from build123d import *

# Parameters (mm, degrees)
SKETCH1_R               = 41.275
SKETCH1_R_2             = 18.6309
BOSS_EXTRUDE1_DEPTH     = 3.81
CUT_EXTRUDE1_DEPTH      = 59.495874641
CUT_EXTRUDE1_DEPTH_BACK = 59.495874641
SKETCH3_R               = 1.049274
CUT_EXTRUDE2_DEPTH      = 59.495874641
CUT_EXTRUDE2_DEPTH_BACK = 59.495874641
SKETCH4_R               = 1.9431


with BuildPart() as part:
    # Sketch1 → Boss-Extrude1 (new body)
    with BuildSketch(Plane(origin=(0, 0, 0), x_dir=(1, 0, 0), z_dir=(0, 1, 0))):
        with Locations(Location((0, 0, 0), (0, 0, 90))):
            Circle(SKETCH1_R)
        with Locations(Location((0, 0, 0), (0, 0, 90))):
            Circle(SKETCH1_R_2, mode=Mode.SUBTRACT)
    extrude(amount=BOSS_EXTRUDE1_DEPTH)

    # Sketch3 → Cut-Extrude1 (cut, two sides: drawn at the far end of the back side and taken through both)
    with BuildSketch(Plane.XZ.offset(-CUT_EXTRUDE1_DEPTH_BACK)):
        with Locations(Location((12.96732128, 21.997045256, 0), (0, 0, 270))):
            Circle(SKETCH3_R)
        with Locations(Location((-12.43267872, 21.997045256, 0), (0, 0, 270))):
            Circle(SKETCH3_R)
        with Locations(Location((-25.13267872, 0, 0), (0, 0, 270))):
            Circle(SKETCH3_R)
        with Locations(Location((-12.43267872, -21.997045256, 0), (0, 0, 270))):
            Circle(SKETCH3_R)
        with Locations(Location((12.96732128, -21.997045256, 0), (0, 0, 270))):
            Circle(SKETCH3_R)
        with Locations(Location((25.66732128, 0, 0), (0, 0, 270))):
            Circle(SKETCH3_R)
    extrude(amount=CUT_EXTRUDE1_DEPTH + CUT_EXTRUDE1_DEPTH_BACK, mode=Mode.SUBTRACT)

    # Sketch4 → Cut-Extrude2 (cut, two sides: drawn at the far end of the back side and taken through both)
    with BuildSketch(Plane(origin=(0, 3.81, 0), x_dir=(1, 0, 0), z_dir=(0, 1, 0)).offset(-CUT_EXTRUDE2_DEPTH_BACK)):
        with Locations(Location((-10.031528943, 32.5374, 0), (0, 0, 270))):
            Circle(SKETCH4_R)
        with Locations(Location((-10.031528943, -32.5374, 0), (0, 0, 270))):
            Circle(SKETCH4_R)
        with Locations(Location((10.031528943, -32.5374, 0), (0, 0, 270))):
            Circle(SKETCH4_R)
        with Locations(Location((10.031528943, 32.5374, 0), (0, 0, 270))):
            Circle(SKETCH4_R)
    extrude(amount=CUT_EXTRUDE2_DEPTH + CUT_EXTRUDE2_DEPTH_BACK, mode=Mode.SUBTRACT)


solid = part.part
Work out the finished part from the listing and answer in its coordinate system (mm). Round coordinates to 2 decimals unless told otherwise and drop trailing zeros. Write each loop counter-clockwise with the first axis right and the second up, starting at its lowest first coordinate (ties: lowest second). Pieces come first, ordered by that corner, then holes. Notation, with made-up numbers: (77, 82) - (103, 82) arc R33 ccw to (103, 110) - close; hole circle Ø9 at (18, 76). An arc over 180 degrees is marked (long way). Answer in a Markdown table with one row per item. Add a question column.
1. A cutting plane is placed at C-C, the plane z = -13. Determine the outline of the cut face in (x, y), and give its area (3 significant figures).
2. A cutting plane is placed at D-D, the plane y = 1.3. Count the separate pieces of the cut face and the enclosed holes in it, and give its area (3 significant figures).
3. A cutting plane is placed at A-A, the plane x = 0. Determine the outline of the cut face in (y, z) (3 decimals), and give its area (3 significant figures).
4. Given pin 1 (1 mm diameter, centred on y = 1.5, z = 4, fed in from -X); pin 2 (2 mm diameter, centred on y = 3, z = -17.5, fed in from +X); pin 3 (1.5 mm diameter, centred on y = 2.5, z = -26, fed in from +X), each flat-ended and moving along its own axis, determine where each tip first touches the part or whether it passes through.
5. A cutting plane is placed at B-B, the plane z = 0. Determine the outline of the cut face in (x, y) (3 decimals), and give its area (3 significant figures).
6. Find the intervals of material crossed by line 1 along X through (y, z) = (2.8, 0) (3 decimals); line 2 along X through (y, z) = (1.75, -22.5); line 3 along Z through (x, y) = (26.5, 0.9), in increasing order. Write a range as from..to.
7. The mould has two halves that part along X. Classify faces 1 (the cylindrical face through (-12.83, 1.93, -22.97)), 2 (the cylindrical face through (-40.924, 1.878, 5.373)), 3 (the flat face through (9, 0, -18)): +X half, -X half, draft (parallel to the pull), parting line (faces both ways), or undercut.
Worked out:
| question | item | result |
|---|---|---|
| 1 | outline | (-39.17, 0) - (-13.35, 0) - (-13.35, 3.81) - (-39.17, 3.81) - close; (13.35, 0) - (39.17, 0) - (39.17, 3.81) - (13.35, 3.81) - close |
| 1 | area | 197 mm^2 |
| 2 | separate pieces | 1 |
| 2 | enclosed holes | 11 |
| 2 | area | 4,190 mm^2 |
| 3 | outline | (0, -41.275) - (3.81, -41.275) - (3.81, -18.631) - (0, -18.631) - close; (0, 18.631) - (3.81, 18.631) - (3.81, 41.275) - (0, 41.275) - close |
| 3 | area | 173 mm^2 |
| 4 | pin 1 | x = -41.13 |
| 4 | pin 2 | x = 37.83 |
| 4 | pin 3 | x = 32.65 |
| 5 | outline | (-41.275, 0) - (-26.182, 0) - (-26.182, 3.81) - (-41.275, 3.81) - close; (-24.083, 0) - (-18.631, 0) - (-18.631, 3.81) - (-24.083, 3.81) - close; (18.631, 0) - (24.618, 0) - (24.618, 3.81) - (18.631, 3.81) - close; (26.717, 0) - (41.275, 0) - (41.275, 3.81) - (26.717, 3.81) - close |
| 5 | area | 157 mm^2 |
| 6 | line 1 | -41.275..-26.182, -24.083..-18.631, 18.631..24.618, 26.717..41.275 |
| 6 | line 2 | -34.6..-13.35, -11.51..12.05, 13.89..34.6 |
| 6 | line 3 | -31.64..-0.64, 0.64..31.64 |
| 7 | face 1 | undercut |
| 7 | face 2 | parting line |
| 7 | face 3 | draft |
